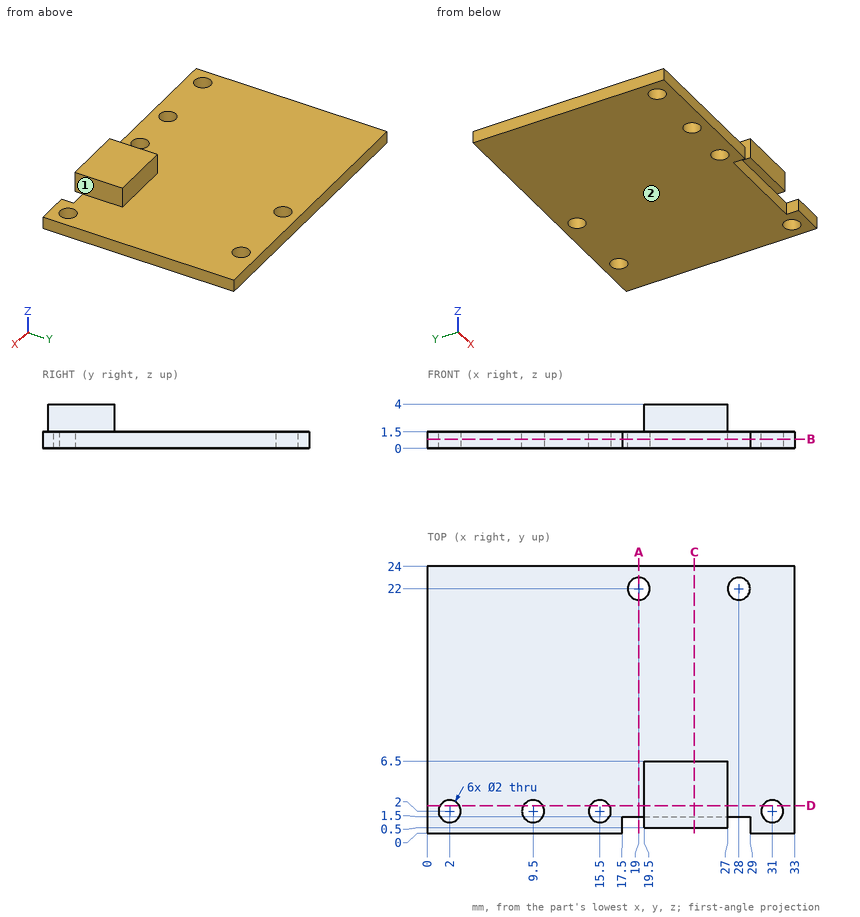
Design review of the part shown in the three views and the two pictorial views. Dimensions are in mm from the part's minimum x, y and z. A direction names the side the tool comes from. Round coordinates to 2 decimals unless told otherwise and drop trailing zeros. Loops run counter-clockwise (first coordinate to the right, second up) from the corner with the lowest first, then second, coordinate; pieces in that order, holes last. Notation, with made-up numbers: (-31.5, 52.5) - (-1.5, 52.5) arc R24 cw to (-1.5, 63.5) - close; hole circle Ø4 at (72, 75.25). An arc over 180 degrees is marked (long way). Use one line per item in the form item = value.
1) We need section D-D on y = 2.5. Write out the cut boundary in (x, z).
Solutions:
outline = (0, 0) - (1.13, 0) - (1.13, 1.5) - (0, 1.5) - close; (2.87, 0) - (8.63, 0) - (8.63, 1.5) - (2.87, 1.5) - close; (10.37, 0) - (14.63, 0) - (14.63, 1.5) - (10.37, 1.5) - close; (16.37, 0) - (30.13, 0) - (30.13, 1.5) - (27, 1.5) - (27, 4) - (19.5, 4) - (19.5, 1.5) - (16.37, 1.5) - close; (31.87, 0) - (33, 0) - (33, 1.5) - (31.87, 1.5) - close
2) We need section A-A on x = 19. Write out the cut boundary in (y, z), then the cut area to 4 significant figures.
Solutions:
outline = (1.5, 0) - (21, 0) - (21, 1.5) - (1.5, 1.5) - close; (23, 0) - (24, 0) - (24, 1.5) - (23, 1.5) - close
area = 30.75 mm2
3) We need section C-C on x = 24. Write out the cut boundary in (y, z), then the cut area to 4 significant figures.
Solutions:
outline = (0.5, 1.5) - (1.5, 1.5) - (1.5, 0) - (24, 0) - (24, 1.5) - (6.5, 1.5) - (6.5, 4) - (0.5, 4) - close
area = 48.75 mm2
4) Wall thickness on probe 1 along Y at (x, z) = (2, 0.8); probe 2 along Z at (x, y) = (11, 4); probe 3 along Y at (x, z) = (22, 1.4): over which ranges is each line inside the solid? List them lowest first.
Solutions:
probe_1 = 0 to 1, 3 to 24
probe_2 = 0 to 1.5
probe_3 = 1.5 to 24
5) We need section B-B on z = 0.85. Write out the cut boundary in (x, y), then the cut area to 3 significant figures.
Solutions:
outline = (0, 0) - (17.5, 0) - (17.5, 1.5) - (29, 1.5) - (29, 0) - (33, 0) - (33, 24) - (0, 24) - close; hole circle Ø2 at (2, 2); hole circle Ø2 at (9.5, 2); hole circle Ø2 at (15.5, 2); hole circle Ø2 at (19, 22); hole circle Ø2 at (28, 22); hole circle Ø2 at (31, 2)
area = 756 mm2
6) Tool access review of the marked faces 1 and 2: name each direction out of +Z, -Z, +X, -X, +Y, -Y from which nothing blocks a thin tool from reaching the whole face with its end or side.
Solutions:
face_1 = +Z, +X, +Y, -Y
face_2 = -Z, +X, -X, +Y, -Y
7) Clearance check with flat-ended pins moving along their axes: P1, Ø1.5, axis at x = 6.5, z = 3, coming from the +Y side; P2, Ø2.5, axis at x = 9.5, y = 2, coming from the +Z side; P3, Ø1.2, axis at x = 25, z = 3.5, coming from the +Y side; P4, Ø1.2, axis at x = 24.5, z = 2.5, coming from the -Y side. State where each tip first meets the part, or that it passes through.
Solutions:
P1 = through
P2 = 1.5
P3 = 6.5
P4 = 0.5
